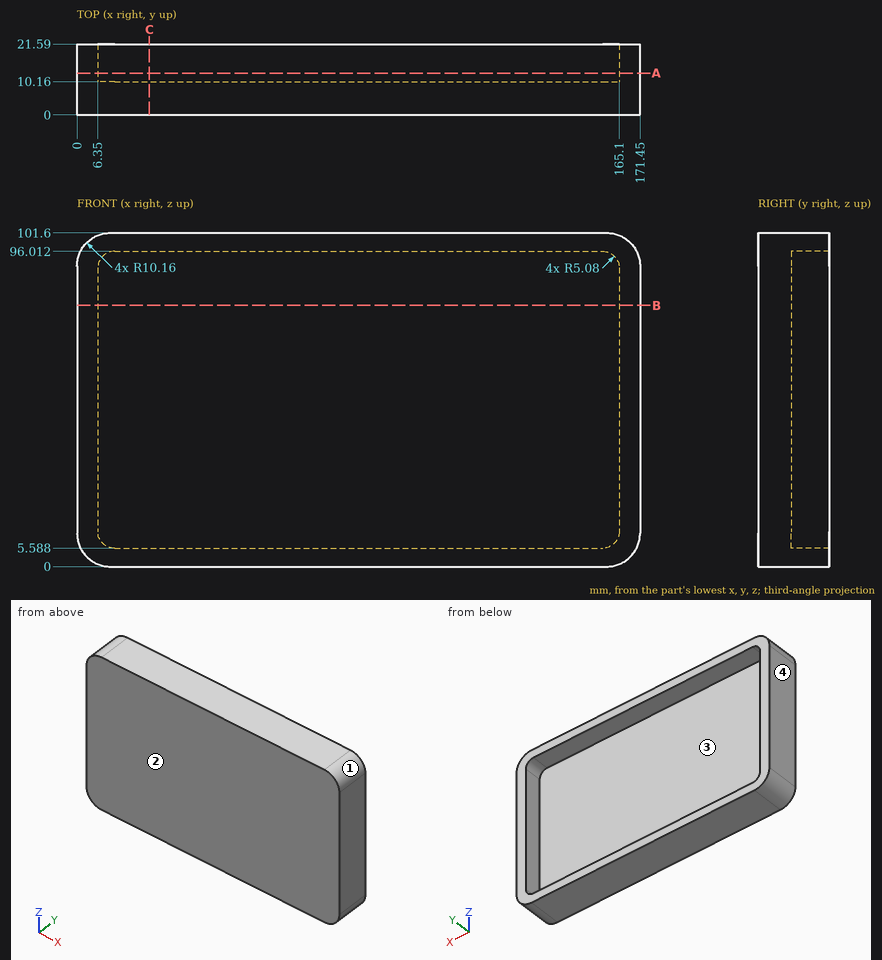
Design review of the part shown in the three views and the two pictorial views. Dimensions are in mm from the part's minimum x, y and z. Round coordinates to 2 decimals unless told otherwise and drop trailing zeros. Order: outer loops, then holes, each group sorted by start corner. A loop starts at its lowest first (then second) coordinate and runs counter-clockwise, first axis right, second up.
Item 1: Add section B-B, the plane z = 79.5. State the section outline as (x, y) points, and give its area (3 significant figures).
Working result:
outline: (0, 0) - (171.45, 0) - (171.45, 21.59) - (165.1, 21.59) - (165.1, 10.16) - (6.35, 10.16) - (6.35, 21.59) - (0, 21.59) - close
area: 1,890 mm2
Item 2: For pin 1 (5.5 mm diameter, centred on x = 104, y = 17.5, fed in from -Z); pin 2 (10 mm diameter, centred on x = 29.5, z = 53.5, fed in from +Y), all flat-tipped, find the tip position at first contact; note any pin that passes through.
Working result:
pin 1: stops at z = 0
pin 2: stops at y = 10.16
Item 3: Add section A-A, the plane y = 12.75. State the section outline as (x, z) points, and give its area (3 significant figures).
Working result:
outline: (0, 10.16) arc R10.16 ccw to (10.16, 0) - (161.29, 0) arc R10.16 ccw to (171.45, 10.16) - (171.45, 91.44) arc R10.16 ccw to (161.29, 101.6) - (10.16, 101.6) arc R10.16 ccw to (0, 91.44) - close; hole (6.35, 10.67) arc R5.08 ccw to (11.43, 5.59) - (160.02, 5.59) arc R5.08 ccw to (165.1, 10.67) - (165.1, 90.93) arc R5.08 ccw to (160.02, 96.01) - (11.43, 96.01) arc R5.08 ccw to (6.35, 90.93) - close
area: 3,000 mm2
Item 4: Add section C-C, the plane x = 22. State the section outline as (y, z) points, and give its area (3 significant figures).
Working result:
outline: (0, 0) - (21.59, 0) - (21.59, 5.59) - (10.16, 5.59) - (10.16, 96.01) - (21.59, 96.01) - (21.59, 101.6) - (0, 101.6) - close
area: 1,160 mm2
Item 5: Draft analysis for pull direction X (two halves, no side actions). For the marked faces 1, 2, 3 and 4, state which applies: released by +X, released by -X, zero draft, split by the parting line, or undercut.
Working result:
face 1: released by +X
face 2: zero draft
face 3: undercut
face 4: released by -X
Item 6: To check wall thickness, follow probe 1 along Z at (x, y) = (135, 19.25); probe 2 along X at (y, z) = (17, 66.5); probe 3 along Y at (x, z) = (22.5, 43). State the ranges of each line that lie inside material, in increasing order.
Working result:
probe 1: z = 0 to 5.59, 96.01 to 101.6
probe 2: x = 0 to 6.35, 165.1 to 171.45
probe 3: y = 0 to 10.16
